```python
from build123d import *

# Parameters (mm, degrees)
F1_DEPTH = 6.35


with BuildPart() as f1:
    # F0 (on Front) → F1 (new body, symmetric)
    with BuildSketch(Plane.XZ):
        with BuildLine():
            Line((63.5, -6.35), (63.5, -9.525))
            Line((63.5, -9.525), (50.0146570307, -9.525))
            ThreePointArc((50.0146570307, -9.525), (68.4968533887, -15.7356778123), (80.01, 0))
            ThreePointArc((80.01, 0), (68.4968533887, 15.7356778123), (50.0146570307, 9.525))
            Line((50.0146570307, 9.525), (63.5, 9.525))
            Line((63.5, 9.525), (63.5, 6.35))
            ThreePointArc((63.5, 6.35), (67.9901280605, 4.4901280605), (69.85, 0))
            ThreePointArc((69.85, 0), (67.9901280605, -4.4901280605), (63.5, -6.35))
        make_face()
        with BuildLine():
            Line((50.0146570307, -9.525), (63.5, -9.525))
            Line((63.5, -9.525), (63.5, -6.35))
            ThreePointArc((63.5, -6.35), (57.15, 0), (63.5, 6.35))
            Line((63.5, 6.35), (63.5, 9.525))
            Line((63.5, 9.525), (50.0146570307, 9.525))
            ThreePointArc((50.0146570307, 9.525), (46.99, 0), (50.0146570307, -9.525))
        make_face()
        with BuildLine():
            Line((-50.0146570307, -9.525), (50.0146570307, -9.525))
            ThreePointArc((50.0146570307, -9.525), (46.99, 0), (50.0146570307, 9.525))
            Line((50.0146570307, 9.525), (-50.0146570307, 9.525))
            ThreePointArc((-50.0146570307, 9.525), (-47.7643221877, 4.9968533887), (-46.99, 0))
            ThreePointArc((-46.99, 0), (-47.7643221877, -4.9968533887), (-50.0146570307, -9.525))
        make_face()
        with BuildLine():
            ThreePointArc((-50.0146570307, 9.525), (-80.01, 0), (-50.0146570307, -9.525))
            Line((-50.0146570307, -9.525), (-63.5, -9.525))
            Line((-63.5, -9.525), (-63.5, -6.35))
            ThreePointArc((-63.5, -6.35), (-69.85, 0), (-63.5, 6.35))
            Line((-63.5, 6.35), (-63.5, 9.525))
            Line((-63.5, 9.525), (-50.0146570307, 9.525))
        make_face()
        with BuildLine():
            Line((-63.5, -9.525), (-50.0146570307, -9.525))
            ThreePointArc((-50.0146570307, -9.525), (-47.7643221877, -4.9968533887), (-46.99, 0))
            ThreePointArc((-46.99, 0), (-47.7643221877, 4.9968533887), (-50.0146570307, 9.525))
            Line((-50.0146570307, 9.525), (-63.5, 9.525))
            Line((-63.5, 9.525), (-63.5, 6.35))
            ThreePointArc((-63.5, 6.35), (-59.0098719395, 4.4901280605), (-57.15, 0))
            ThreePointArc((-57.15, 0), (-59.0098719395, -4.4901280605), (-63.5, -6.35))
            Line((-63.5, -6.35), (-63.5, -9.525))
        make_face()
    extrude(amount=F1_DEPTH, both=True)


solid = f1.part
```
The listing builds one solid part. Answer for the finished solid, in the listing's coordinates (mm). A direction names the side the tool comes from. Coordinates: 2 decimals unless noted, no trailing zeros. Order: outer loops, then holes, each group sorted by start corner. A loop starts at its lowest first (then second) coordinate and runs counter-clockwise, first axis right, second up. Notation, with made-up numbers: M -27,77 L 26,77 A27 ccw 26,101 Z; hole C 71.25,84 d3. An arc over 180 degrees is marked long. Answer as a JSON object with one key per item and string values. Group by question number.
1. Section D-D on x = -15.5 is taken. Write down the section's boundary in (y, z) (3 decimals).
2. A tool of negligible diameter and unlimited length cuts with its end or side. For faces 3 (the cylindrical face through (80, -0.1, -0.6)), 4 (the flat face through (1, 0, 9.525)), from which of +Z, -Z, +X, -X, +Y, -Y can it reach the whole face along a straight path? Write none if from no direction.
3. Flat-ended cylindrical pins translate along their axes: P1, Ø5, axis at y = -0.5, z = 5, coming from the -X side; P2, Ø2, axis at y = -1, z = 0.5, coming from the -X side; P3, Ø1.5, axis at y = 1, z = -2.5, coming from the -X side; P4, Ø6.5, axis at x = -22.5, y = 2, coming from the -Z side (3 decimals). Find the tip coordinate at first contact, or state that the pin passes through.
4. Section B-B on z = 11 is taken. Write down the section's boundary in (x, y).
5. Straight lines are drawn through the part: line 1 (Z direction, x = -63.5, y = -0.5); line 2 (X direction, y = -4, z = -3); line 3 (X direction, y = 5.75, z = 2.5). For each, find the intervals that lie inside material, in ascending order.
6. Section C-C on z = 2 is taken. Write down the section's boundary in (x, y), then the cut area to 3 significant figures.
7. Determine the mould class of faces 1 (the flat face through (-1, 0, -9.525)), 2 (the flat face through (-1, -6.35, 0)) for opening direction X: released by +X, released by -X, zero draft, split by the parting line, or undercut.
8. Section A-A on y = -4.75 is taken. Write down the section's boundary in (x, z) (3 decimals).
Values follow:
{
 "1": {"outline": "M -6.35,-9.525 L 6.35,-9.525 L 6.35,9.525 L -6.35,9.525 Z"},
 "2": {"face 3": "+Y, -Y", "face 4": "+Z, +Y, -Y"},
 "3": {"P1": "x = -79.82", "P2": "x = -80.01", "P3": "x = -79.92", "P4": "z = -9.525"},
 "4": {"outline": "M -75.81,-6.35 L -51.19,-6.35 L -51.19,6.35 L -75.81,6.35 Z; M 51.19,-6.35 L 75.81,-6.35 L 75.81,6.35 L 51.19,6.35 Z"},
 "5": {"line 1": "-16.51 to -6.35, 6.35 to 16.51", "line 2": "-79.74 to -69.1, -57.9 to 57.9, 69.1 to 79.74", "line 3": "-79.82 to -69.34, -57.66 to 57.66, 69.34 to 79.82"},
 "6": {"outline": "M -79.89,-6.35 L -69.53,-6.35 L -69.53,6.35 L -79.89,6.35 Z; M -57.47,-6.35 L 57.47,-6.35 L 57.47,6.35 L -57.47,6.35 Z; M 69.53,-6.35 L 79.89,-6.35 L 79.89,6.35 L 69.53,6.35 Z", "area": "1,720 mm2"},
 "7": {"face 1": "undercut", "face 2": "zero draft"},
 "8": {"outline": "M -50.015,-9.525 L 50.015,-9.525 A16.51 ccw long 50.015,9.525 L -50.015,9.525 A16.51 ccw long Z; hole C -63.5,0 d12.7; hole C 63.5,0 d12.7"}
}
